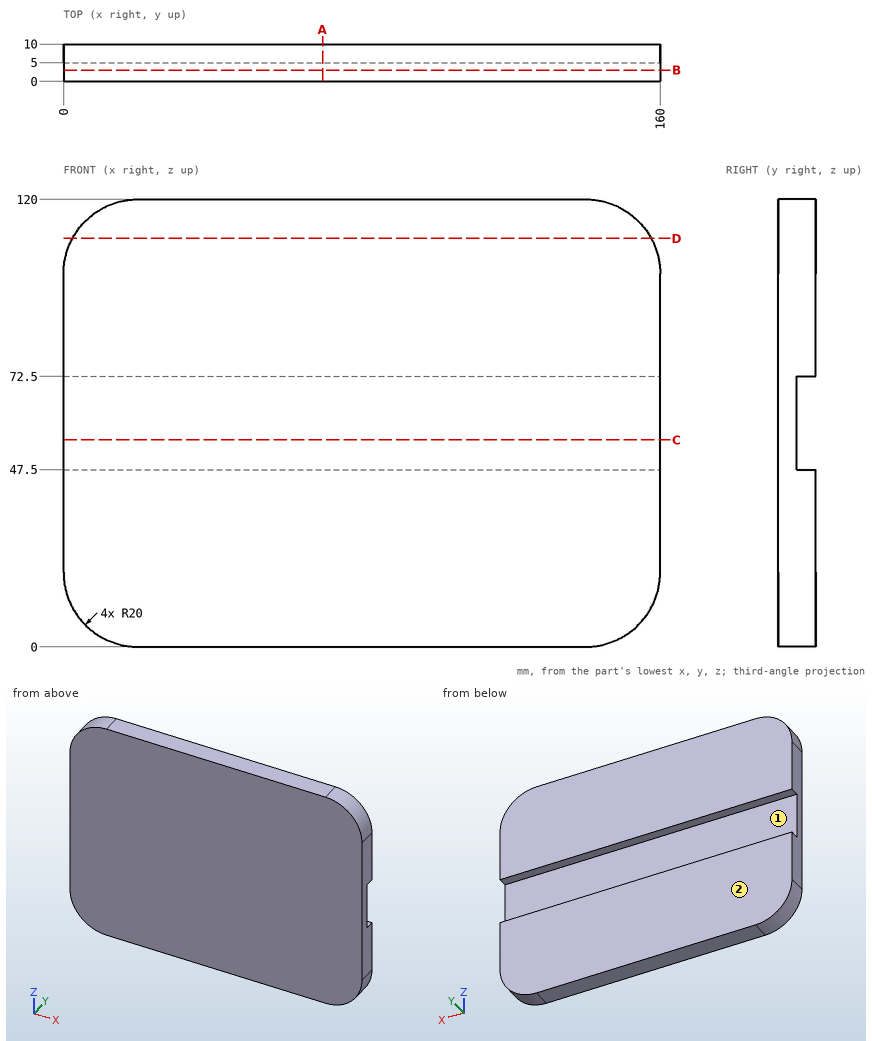
Part print with two shaded views. Sizes in mm from the minimum x, y, z corner. Coordinates: 2 decimals unless noted, no trailing zeros. Order: outer loops, then holes, each group sorted by start corner. A loop starts at its lowest first (then second) coordinate and runs counter-clockwise, first axis right, second up. Notation, with made-up numbers: M 64.5,33.5 L 121.5,33.5 A23 cw 121.5,63.5 Z; hole C 24,-26 d10. An arc over 180 degrees is marked long. One line per question, with ' | ' between items. Start each with the question number.
1. Cut at C-C (z = 55.5). Write the cut outline in (x, y), plus the area to 3 significant figures.
2. Flat gauge pin, fed straight in: P1, Ø20, axis at x = 76, z = 58, coming from the +Y side. Where does the tip first touch, or does it go through?
3. Cut at B-B (y = 3). Write the cut outline in (x, z), plus the area to 3 significant figures.
4. Cut at D-D (z = 109.5). Write the cut outline in (x, y), plus the area to 3 significant figures.
5. Cut at A-A (x = 69.5). Write the cut outline in (y, z).
6. Mould opens along Z. For the marked faces 1 and 2 say: +Z half, -Z half, draft (parallel to the pull), parting line (faces both ways), or undercut.
7. Wall check: line 1 along Z through (x, y) = (108.5, 6.75); line 2 along Y through (x, z) = (46, 65.5); line 3 along X through (y, z) = (2.25, 103.5). Give the ranges that are in metal, low to high. Write a range as [from, to].
The answers:
1) outline: M 0,0 L 160,0 L 160,5 L 0,5 Z | area: 800 mm2
2) P1: stops at y = 5
3) outline: M 0,20 A20 ccw 20,0 L 140,0 A20 ccw 160,20 L 160,100 A20 ccw 140,120 L 20,120 A20 ccw 0,100 Z | area: 18,900 mm2
4) outline: M 2.4,0 L 157.6,0 L 157.6,10 L 2.4,10 Z | area: 1,550 mm2
5) outline: M 0,0 L 10,0 L 10,47.5 L 5,47.5 L 5,72.5 L 10,72.5 L 10,120 L 0,120 Z
6) face 1: undercut | face 2: draft
7) line 1: z = [0, 47.5], [72.5, 120] | line 2: y = [0, 5] | line 3: x = [0.31, 159.69]
